from build123d import *

# Parameters (mm, degrees)
SKETCH_1_R          = 21.25
SKETCH_1_R_2        = 4.75
SKETCH_1_R_3        = 1.5
EXTRUDE_1_DEPTH     = 31
SKETCH_1_3_R        = 1.5
CUT_EXTRUDE_1_DEPTH = 5


with BuildPart() as part:
    # Sketch 1 → Extrude 1 (new body)
    with BuildSketch(Plane(origin=(0, 0, 0), x_dir=(1, 0, 0), z_dir=(0, 1, 0))):
        with Locations(Location((0, 0, 0), (0, 0, 270))):
            Circle(SKETCH_1_R)
        with Locations(Location((0, 0, 0), (0, 0, 270))):
            Circle(SKETCH_1_R_2, mode=Mode.SUBTRACT)
        with Locations(Location((0, 13.5, 0), (0, 0, 270))):
            Circle(SKETCH_1_R_3, mode=Mode.SUBTRACT)
        with Locations(Location((11.691342951, -6.75, 0), (0, 0, 270))):
            Circle(SKETCH_1_R_3, mode=Mode.SUBTRACT)
        with Locations(Location((-11.691342951, -6.75, 0), (0, 0, 270))):
            Circle(SKETCH_1_R_3, mode=Mode.SUBTRACT)
    extrude(amount=EXTRUDE_1_DEPTH)

    # Sketch 1_3 → Cut-Extrude 1 (cut)
    with BuildSketch(Plane(origin=(0, 0, 0), x_dir=(1, 0, 0), z_dir=(0, 1, 0))):
        with Locations(Location((10.522208656, 6.075, 0), (0, 0, 270))):
            Circle(SKETCH_1_3_R)
        with Locations(Location((0, -12.15, 0), (0, 0, 270))):
            Circle(SKETCH_1_3_R)
        with Locations(Location((-10.522208656, 6.075, 0), (0, 0, 270))):
            Circle(SKETCH_1_3_R)
    extrude(amount=CUT_EXTRUDE_1_DEPTH, mode=Mode.SUBTRACT)


solid = part.part
Model file for the job. Use its own axes, mm. A direction names the side the tool comes from. Give positions to 0.01 mm unless a question says otherwise; leave off trailing zeros. Loops run counter-clockwise (first coordinate to the right, second up) from the corner with the lowest first, then second, coordinate; pieces in that order, holes last.
Item 1: Drop flat-ended pins along their axis: P1, Ø10, axis at x = 9, y = 14, coming from the +Z side; P2, Ø1.5, axis at x = -0.5, z = 12.5, coming from the -Y side; P3, Ø2, axis at x = -1, y = 13, coming from the +Z side; P4, Ø1, axis at x = 13.5, y = 8, coming from the -Z side. Give the stop position or say it passes through.
Check values:
P1: stops at z = 20.87
P2: stops at y = 5
P3: stops at z = 21.25
P4: stops at z = -16.81
Item 2: Slice it at C-C (z = 6.75). Write the cut outline in (x, y), plus the area to 3 significant figures.
Check values:
outline: (-20.15, 0) - (-13.19, 0) - (-13.19, 31) - (-20.15, 31) - close; (-10.19, 0) - (10.19, 0) - (10.19, 31) - (-10.19, 31) - close; (13.19, 0) - (20.15, 0) - (20.15, 31) - (13.19, 31) - close
area: 1,060 mm2
Item 3: Mould opens along Z. For faces 1 (the face through (0, 15, -15)), 2 (the face through (-12.93, 15.283, -16.863)), 3 (the face through (5, 0, 0)) say: +Z half, -Z half, draft (parallel to the pull), parting line (faces both ways), or undercut.
Check values:
face 1: undercut
face 2: parting line
face 3: draft
Item 4: Drill centre lines: line 1 along X through (y, z) = (23, 6); line 2 along Z through (x, y) = (13, 15.5); line 3 along Z through (x, y) = (0.5, 22). Where is each one in solid material? Low to high.
Check values:
line 1: x = -20.39 to -12.99, -10.39 to 10.39, 12.99 to 20.39
line 2: z = -16.81 to 6.02, 7.48 to 16.81
line 3: z = -21.24 to -14.91, -12.09 to -4.72, 4.72 to 21.24
Item 5: Slice it at A-A (x = 0). Write the cut outline in (y, z).
Check values:
outline: (0, -21.25) - (31, -21.25) - (31, -15) - (0, -15) - close; (0, -12) - (31, -12) - (31, -4.75) - (0, -4.75) - close; (0, 4.75) - (31, 4.75) - (31, 21.25) - (0, 21.25) - (0, 13.65) - (5, 13.65) - (5, 10.65) - (0, 10.65) - close
Item 6: Slice it at D-D (y = 4). Write the cut outline in (x, z) (3 decimals).
Check values:
outline: circle Ø42.5 at (0, 0); hole circle Ø3 at (-11.691, 6.75); hole circle Ø3 at (-10.522, -6.075); hole circle Ø9.5 at (0, 0); hole circle Ø3 at (0, -13.5); hole circle Ø3 at (0, 12.15); hole circle Ø3 at (10.522, -6.075); hole circle Ø3 at (11.691, 6.75)
Item 7: Which spindle directions (+Z, -Z, +X, -X, +Y, -Y) get a long thin tool onto all of the face, cutting with end or side? Do faces 4 (the face through (0, 5, 12)), 5 (the face through (10.78, 15.28, 5.56)). Say none if no direction does.
Check values:
face 4: -Y
face 5: +Y, -Y
Item 8: Slice it at B-B (z = 2). Write the cut outline in (x, y), plus the area to 3 significant figures.
Check values:
outline: (-21.16, 0) - (-4.31, 0) - (-4.31, 31) - (-21.16, 31) - close; (4.31, 0) - (21.16, 0) - (21.16, 31) - (4.31, 31) - close
area: 1,040 mm2
